Source: three-view drawing plus pictorial views. Frame: mm from the lowest corner of the part. A direction names the side the tool comes from. Give positions to 0.01 mm unless a question says otherwise; leave off trailing zeros. Loops run counter-clockwise (first coordinate to the right, second up) from the corner with the lowest first, then second, coordinate; pieces in that order, holes last. Notation, with made-up numbers: M 89,-2.75 L 143,-2.75 A13 ccw 143,2.25 Z; hole C -0.5,10.5 d9. An arc over 180 degrees is marked long. Write item = value, one per line.
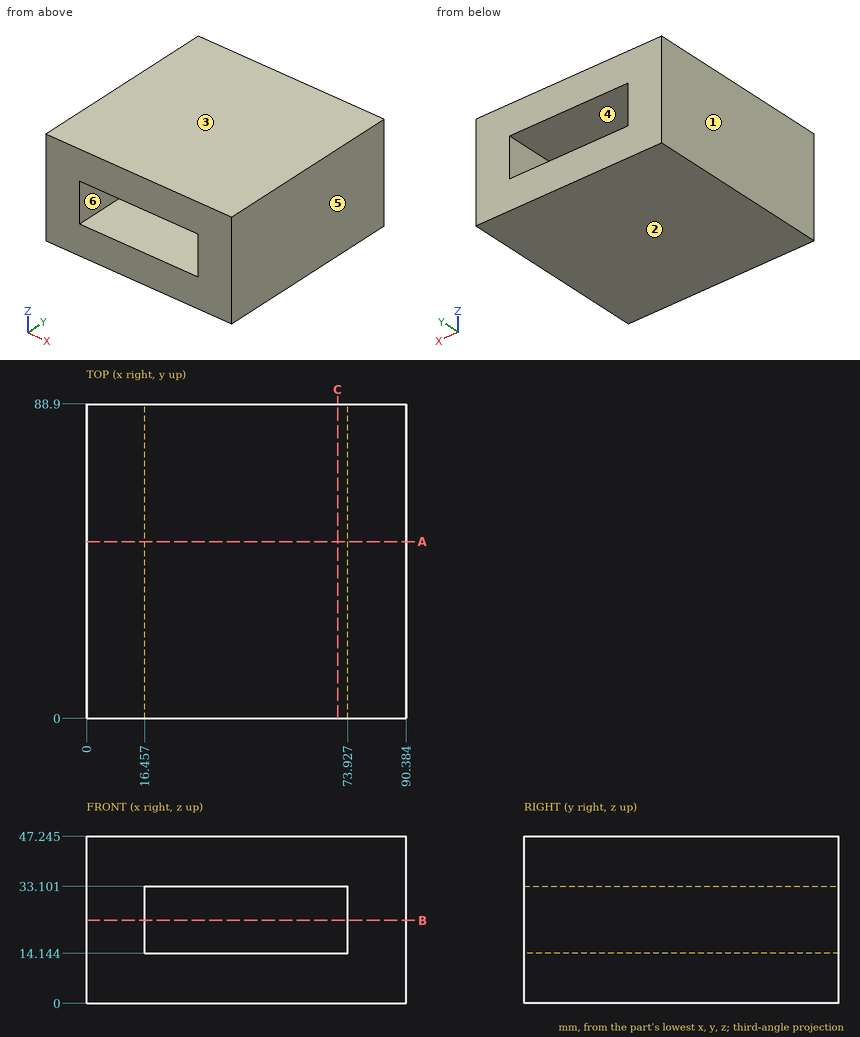
1. First-contact query: pin 1 Ø1.5 at (x, z) = (38.5, 30.5) entering from -Y. Flat tip, straight axial feed; report the tip coordinate or a pass-through.
Derived:
pin_1 = through
2. Pull-direction query (Z, two-part tool) for the marked faces 1, 2, 3 and 4; classes: +Z half, -Z half, draft (parallel to the pull), parting line (faces both ways), or undercut.
Derived:
face_1 = draft
face_2 = -Z half
face_3 = +Z half
face_4 = undercut
3. Cut plane C-C, the plane x = 71. Return the cut outline in (y, z) (1 decimal).
Derived:
outline = M 0,0 L 88.9,0 L 88.9,14.1 L 0,14.1 Z; M 0,33.1 L 88.9,33.1 L 88.9,47.2 L 0,47.2 Z
4. Material intervals for probe 1 along Z at (x, y) = (68, 43) (1 decimal); probe 2 along X at (y, z) = (40.5, 30) (1 decimal), sorted ascending. Write a range as from..to.
Derived:
probe_1 = 0..14.1, 33.1..47.2
probe_2 = 0..16.5, 73.9..90.4
5. Cut plane B-B, the plane z = 23.5. Return the cut outline in (x, y) (1 decimal).
Derived:
outline = M 0,0 L 16.5,0 L 16.5,88.9 L 0,88.9 Z; M 73.9,0 L 90.4,0 L 90.4,88.9 L 73.9,88.9 Z
6. Reachability of the marked faces 5 and 6 from +Z, -Z, +X, -X, +Y, -Y: full face, straight path, thin tool, end or side. Return the list, or none.
Derived:
face_5 = +Z, -Z, +X, +Y, -Y
face_6 = +Y, -Y
7. Cut plane A-A, the plane y = 50. Return the cut outline in (x, z) (1 decimal), then the cut area to 3 significant figures.
Derived:
outline = M 0,0 L 90.4,0 L 90.4,47.2 L 0,47.2 Z; hole M 16.5,14.1 L 73.9,14.1 L 73.9,33.1 L 16.5,33.1 Z
area = 3,180 mm²
